```python
from build123d import *

# Parameters (mm, degrees)
F0_R      = 25
F1_DEPTH  = 25
F2_R      = 5
F1_FACE_R = 20
F3_DEPTH  = 20
F4_R      = 20
F5_DEPTH  = 22.5


with BuildPart() as f1:
    # F0 (on Top) → F1 (new body)
    with BuildSketch(Plane.XY):
        Circle(F0_R)
    extrude(amount=F1_DEPTH)

    # F2
    f2_edges = [f1.edges().sort_by_distance(p)[0] for p in [
        (-25, 0, 25),
    ]]
    fillet(f2_edges, radius=F2_R)

    # F1_face (on face) → F3 (join)
    with BuildSketch(Plane.XY.offset(25)):
        Circle(F1_FACE_R)
    extrude(amount=-F3_DEPTH)

    # F4 (on face) → F5 (cut)
    with BuildSketch(Plane.XY.offset(25)):
        Circle(F4_R)
    extrude(amount=-F5_DEPTH, mode=Mode.SUBTRACT)


solid = f1.part
```
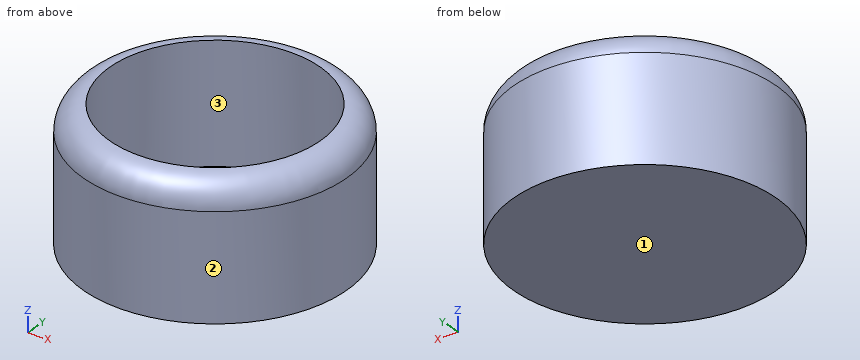
Can you work these out from the model? Positions are in its coordinate system, mm. Face numbers are marked on the shaded views. Round coordinates to 2 decimals unless told otherwise and drop trailing zeros. Loops run counter-clockwise (first coordinate to the right, second up) from the corner with the lowest first, then second, coordinate; pieces in that order, holes last. Notation, with made-up numbers: (20, -40) -> (55, -40) arc R21 cw to (55, -12) -> close; hole circle Ø6 at (-25, 54). An arc over 180 degrees is marked (long way). One line per item, written item: value. Start each with the question number.
1. If we section it at A-A, the plane y = 0: Write out the boundary of the cut face in (x, z), then the cut area to 3 significant figures.
2. For pin 1 (24 mm diameter, centred on x = 0, y = 0, fed in from +Z); pin 2 (12 mm diameter, centred on y = 10.5, z = 6, fed in from +X); pin 3 (6 mm diameter, centred on x = -5.5, z = 20.5, fed in from +Y), each with a flat end and sliding along its axis, tell me the tip position at first contact or that it passes through.
3. If we mould it in two halves opening along Y, with no side actions, what happens to the marked faces 1, 2 and 3? For each: pulls with the +Y half, pulls with the -Y half, needs draft (parallel to the pull), parting line crosses it, or undercut.
4. If I drill on probe 1 along Y at (x, z) = (0, 13.5); probe 2 along Y at (x, z) = (2, 15); probe 3 along X at (y, z) = (18.5, 5.25), over which ranges is the centre line in solid material (lowest first)?
5. If we section it at C-C, the plane z = 5.75: Write out the boundary of the cut face in (x, y).
Calculated:
1. outline: (-25, 0) -> (25, 0) -> (25, 20) arc R5 ccw to (20, 25) -> (20, 2.5) -> (-20, 2.5) -> (-20, 25) arc R5 ccw to (-25, 20) -> close
1. area: 339 mm²
2. pin 1: stops at z = 2.5
2. pin 2: stops at x = 24.59
2. pin 3: stops at y = 24.87
3. face 1: needs draft
3. face 2: parting line crosses it
3. face 3: undercut
4. probe 1: y = -25 to -20, 20 to 25
4. probe 2: y = -24.92 to -19.9, 19.9 to 24.92
4. probe 3: x = -16.82 to -7.6, 7.6 to 16.82
5. outline: circle Ø50 at (0, 0); hole circle Ø40 at (0, 0)
